```python
from build123d import *

# Parameters (mm, degrees)
SKETCH_1_W      = 9
SKETCH_1_H      = 8
EXTRUDE_1_DEPTH = 3.75
SKETCH_2_R      = 2.5
EXTRUDE_2_DEPTH = 3
CHAMFER_1_SIZE  = 0.5
EXTRUDE_3_DEPTH = 0.8
SKETCH_4_R      = 0.75
EXTRUDE_4_DEPTH = 5.8
EXTRUDE_4_DRAFT = -10
FILLET_1_R      = 1.3


with BuildPart() as part:
    # Эскиз1 → Бобышка-Вытянуть1 (new, symmetric)
    with BuildSketch(Plane(origin=(0, 0, 0), x_dir=(1, 0, 0), z_dir=(0, 1, 0))):
        Rectangle(SKETCH_1_W, SKETCH_1_H)
    extrude(amount=EXTRUDE_1_DEPTH, both=True)

    # Эскиз2 → Бобышка-Вытянуть2 (add)
    with BuildSketch(Plane(origin=(0, 3.75, 0), x_dir=(1, 0, 0), z_dir=(0, 1, 0))):
        with Locations(Location((0, 0, 0), (0, 0, 270))):
            Circle(SKETCH_2_R)
    extrude(amount=EXTRUDE_2_DEPTH)

    # Фаска1
    chamfer_1_edges = [part.edges().sort_by_distance(p)[0] for p in [
        (0, 6.75, -2.5),
    ]]
    chamfer(chamfer_1_edges, length=CHAMFER_1_SIZE)

    # Эскиз3 → Бобышка-Вытянуть3 (add)
    with BuildSketch(Plane(origin=(0, 5.65, 0), x_dir=(1, 0, 0), z_dir=(0, 1, 0))):
        with BuildLine():
            Line((-2.020987717, -3.283260181), (2.020987717, -3.283260181))
            ThreePointArc((2.020987717, -3.283260181), (2.728094498, -2.990366962), (3.020987717, -2.283260181))
            Line((3.020987717, -2.283260181), (3.020987717, 2.283260181))
            ThreePointArc((3.020987717, 2.283260181), (2.728094498, 2.990366962), (2.020987717, 3.283260181))
            Line((2.020987717, 3.283260181), (-2.020987717, 3.283260181))
            ThreePointArc((-2.020987717, 3.283260181), (-2.728094498, 2.990366962), (-3.020987717, 2.283260181))
            Line((-3.020987717, 2.283260181), (-3.020987717, -2.283260181))
            ThreePointArc((-3.020987717, -2.283260181), (-2.728094498, -2.990366962), (-2.020987717, -3.283260181))
        make_face()
    extrude(amount=-EXTRUDE_3_DEPTH)


with BuildPart() as extrude_4_tool:
    # Эскиз4 → Бобышка-Вытянуть4 (with draft: the straight prism first)
    with BuildSketch(Plane(origin=(0, 6.75, 0), x_dir=(1, 0, 0), z_dir=(0, 1, 0))):
        Circle(SKETCH_4_R)
    extrude(amount=EXTRUDE_4_DEPTH)
    # Бобышка-Вытянуть4: the draft: its side faces are tilted about the plane it starts from
    extrude_4_sides = [extrude_4_tool.faces().sort_by_distance(p)[0] for p in [
        (-0.75, 9.65, 0),
    ]]
    draft(extrude_4_sides, Plane(origin=(0, 6.75, 0), x_dir=(1, 0, 0), z_dir=(0, 1, 0)), EXTRUDE_4_DRAFT)


with BuildPart() as part_1:
    add(part.part)

    # Бобышка-Вытянуть4: add extrude_4_tool
    add(extrude_4_tool.part)

    # Скругление1
    fillet_1_edges = [part_1.edges().sort_by_distance(p)[0] for p in [
        (-1.772696488, 12.55, 0),
    ]]
    fillet(fillet_1_edges, radius=FILLET_1_R)


solid = part_1.part
```
The model under review builds one solid part; all positions refer to its coordinate system, in mm. A direction names the side the tool comes from. Round coordinates to 2 decimals unless told otherwise and drop trailing zeros. Write each loop counter-clockwise with the first axis right and the second up, starting at its lowest first coordinate (ties: lowest second). Pieces come first, ordered by that corner, then holes. Notation, with made-up numbers: M 39,85.5 L 48,85.5 A9 cw 48,91.5 Z; hole C 50.5,-17.5 d5. An arc over 180 degrees is marked long. Use CSV: the item, a comma, the result in double quotes. Start each with the question number.
(1) Tool access review of faces 1 (the face through (-2.72, 5.26, -3)), 2 (the face through (0, 3.75, -3)), 3 (the face through (2.74, 5.26, -2.98)): name each direction out of +Z, -Z, +X, -X, +Y, -Y from which nothing blocks a thin tool from reaching the whole face with its end or side.
(2) The part is to be moulded in two halves that separate along Y. For faces 4 (the face through (-2, 4.85, -2)), 5 (the face through (-4.5, 0, 0)), 6 (the face through (0, -3.75, 0)), say which applies: +Y half, -Y half, draft (parallel to the pull), parting line (faces both ways), or undercut.
(3) We need section B-B, the plane x = -3.25. State the section outline as (y, z) points, then the cut area to 3 significant figures.
(4) For line 1 along Y through (x, z) = (2.75, -1.5); line 2 along Y through (x, z) = (-3.5, -2.25); line 3 along X through (y, z) = (6, 1.5), list the stretches that pass through material, from the lowest coordinate up.
(5) We need section A-A, the plane z = 2.75. State the section outline as (x, y) points.
(6) Clearance check with flat-ended pins moving along their axes: P1, Ø0.6, axis at y = 5, z = 1, coming from the +X side; P2, Ø0.6, axis at x = -0.5, y = 5.5, coming from the +Z side; P3, Ø0.6, axis at x = 0.5, y = 5, coming from the -Z side. State where each tip first meets the part, or that it passes through.
Findings:
1,face 1,"-Z, -X, +Y"
1,face 2,"none"
1,face 3,"-Z, +X, +Y"
2,face 4,"undercut"
2,face 5,"draft"
2,face 6,"-Y half"
3,outline,"M -3.75,-4 L 3.75,-4 L 3.75,4 L -3.75,4 Z"
3,area,"60.0 mm^2"
4,line 1,"-3.75 to 3.75, 4.85 to 5.65"
4,line 2,"-3.75 to 3.75"
4,line 3,"-2 to 2"
5,outline,"M -4.5,-3.75 L 4.5,-3.75 L 4.5,3.75 L -4.5,3.75 Z; M -2.91,4.85 L 2.91,4.85 L 2.91,5.65 L -2.91,5.65 Z"
6,P1,"x = 3.02"
6,P2,"z = 3.28"
6,P3,"z = -3.28"
